Verification items for the finished model (mm, model axes). Coordinates: 2 decimals unless noted, no trailing zeros. Write each loop counter-clockwise with the first axis right and the second up, starting at its lowest first coordinate (ties: lowest second). Pieces come first, ordered by that corner, then holes. Notation, with made-up numbers: M 27,63.5 L 67,63.5 A34 cw 67,101.5 Z; hole C -20.75,41.25 d10. An arc over 180 degrees is marked long. Answer in a Markdown table with one row per item.
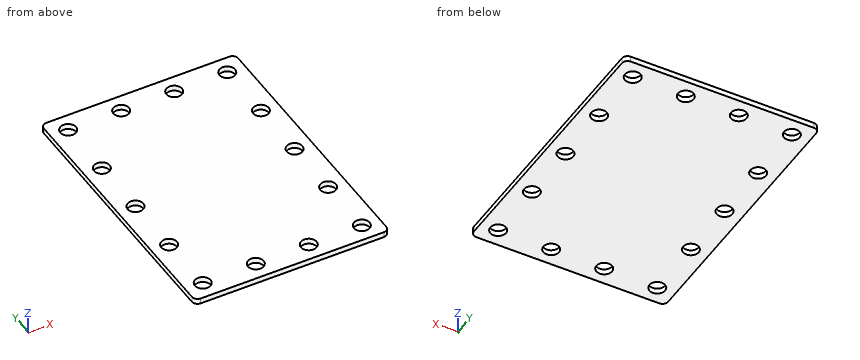
Autodesk Inventor part; units mm, degrees
ref_plane "YZ Plane" through (0, 0, 0) normal (1, 0, 0) x (0, 1, 0)
ref_plane "XZ Plane" through (0, 0, 0) normal (0, 1, 0) x (-1, 0, 0)
ref_plane "XY Plane" through (0, 0, 0) normal (0, 0, 1) x (1, 0, 0)
sketch "Sketch2" plane through (0, 0, 0) normal (0, 0, 1) x (1, 0, 0)
  line L0 (-55, -98) -> (55, -98)
  line L1 (55, -98) -> (55, 98)
  line L2 (55, 98) -> (-55, 98)
  line L3 (-55, 98) -> (-55, -98)
  line L4 (-55, -98) -> (55, 98) construction
  line L5 (55, -98) -> (-55, 98) construction
  line L6 (-105, -148) -> (105, -148)
  line L7 (105, -148) -> (105, 148)
  line L8 (105, 148) -> (-105, 148)
  line L9 (-105, 148) -> (-105, -148)
  point P0 (0, 0)
  dimension "d31" = 50
  dimension "d60" = 196
  dimension "d61" = 110
extrude "Plate2" add sketch "Sketch2" along normal blind 6 contours L3 L2 L1 L0 | L9 L8 L7 L6
sketch "Sketch5" plane through (0, 0, 6) normal (0, 0, 1) x (1, 0, 0)
  line L0 (105, -148) -> (-105, -148) construction
  line L1 (105, 148) -> (105, -148) construction
  line L2 (-105, 148) -> (105, 148) construction
  line L3 (-105, -148) -> (-105, 148) construction
  line L4 (-86, 129) -> (86, 129) construction
  line L5 (86, 129) -> (86, -129) construction
  line L6 (86, -129) -> (-86, -129) construction
  line L7 (-86, -129) -> (-86, 129) construction
  line L8 (-28.6667, -129) -> (28.6667, -129)
  line L9 (28.6667, -129) -> (28.6667, 129) construction
  line L10 (28.6667, 129) -> (-28.6667, 129)
  line L11 (-28.6667, 129) -> (-28.6667, -129) construction
  line L12 (-28.6667, 0) -> (28.6667, 0) construction
  point P0 (0, 0)
  point P1 (0, -129)
  point P2 (-86, -64.5)
  point P3 (-86, 0)
  point P4 (-86, 64.5)
  point P5 (86, 64.5)
  point P6 (86, 0)
  point P7 (86, -64.5)
  point P8 (0, 0)
  dimension "d34" = 19
  dimension "d47" = 64.5
  dimension "d48" = 64.5
  dimension "d49" = 57.3333
  dimension "d50" = 57.3333
fillet "Corner Round1" radius 6 4 edges at (-105, -148, 3) (-105, 148, 3) (105, 148, 3) (105, -148, 3)
hole "Hole1" at (-86, -129, 6) at (-86, -64.5, 6) at (-86, 0, 6) at (-86, 64.5, 6) at (-86, 129, 6) at (86, 129, 6) at (86, 64.5, 6) at (86, 0, 6) at (86, -64.5, 6) at (86, -129, 6) at (-28.6667, -129, 6) at (28.6667, 129, 6) at (28.6667, -129, 6) at (-28.6667, 129, 6) direction (0, 0, -1) diameter 17 end through all
equation "\"d60\" = ChargingHatch_width - 2 * Thickness"
equation "\"d61\" = ChargingHatch_hight - 2 * Thickness"
equation "\"d56\" = Thickness"
equation "\"d14\" = Thickness"
equation "\"BendReliefWidth\" = Thickness"
equation "\"BendReliefDepth\" = 0.5 * Thickness"
equation "\"CornerReliefSize\" = 4 * Thickness"
equation "\"MinimumRemnant\" = 2 * Thickness"
equation "\"TransitionRadius\" = BendRadius"
equation "\"JacobiRadiusSize\" = BendRadius"
equation "\"GapSize\" = Thickness"
properties part number "PRS 9607 charging flange rect_D1200" material "Steel"
1) Thickness scan on L1, parallel to Y at x = -29, z = 2.7; L2, parallel to X at y = 129, z = 2.2; L3, parallel to X at y = 64.5, z = 2. Record the ranges inside material, lowest first. Write a range as [from, to].
Response values:
| item | result |
|---|---|
| L1 | y = [-148, -137.49], [-120.51, 120.51], [137.49, 148] |
| L2 | x = [-105, -94.5], [-77.5, -37.17], [-20.17, 20.17], [37.17, 77.5], [94.5, 105] |
| L3 | x = [-105, -94.5], [-77.5, 77.5], [94.5, 105] |
2) Sectioned sample at A-A (y = -64.5). Record the cut outline in (x, z).
Response values:
| item | result |
|---|---|
| outline | M -105,0 L -94.5,0 L -94.5,6 L -105,6 Z; M -77.5,0 L 77.5,0 L 77.5,6 L -77.5,6 Z; M 94.5,0 L 105,0 L 105,6 L 94.5,6 Z |
3) Sectioned sample at D-D (x = 24.5). Record the cut outline in (y, z).
Response values:
| item | result |
|---|---|
| outline | M -148,0 L -136.41,0 L -136.41,6 L -148,6 Z; M -121.59,0 L 121.59,0 L 121.59,6 L -121.59,6 Z; M 136.41,0 L 148,0 L 148,6 L 136.41,6 Z |
4) Sectioned sample at C-C (y = -129). Record the cut outline in (x, z).
Response values:
| item | result |
|---|---|
| outline | M -105,0 L -94.5,0 L -94.5,6 L -105,6 Z; M -77.5,0 L -37.17,0 L -37.17,6 L -77.5,6 Z; M -20.17,0 L 20.17,0 L 20.17,6 L -20.17,6 Z; M 37.17,0 L 77.5,0 L 77.5,6 L 37.17,6 Z; M 94.5,0 L 105,0 L 105,6 L 94.5,6 Z |
5) Sectioned sample at B-B (x = 86). Record the cut outline in (y, z).
Response values:
| item | result |
|---|---|
| outline | M -148,0 L -137.5,0 L -137.5,6 L -148,6 Z; M -120.5,0 L -73,0 L -73,6 L -120.5,6 Z; M -56,0 L -8.5,0 L -8.5,6 L -56,6 Z; M 8.5,0 L 56,0 L 56,6 L 8.5,6 Z; M 73,0 L 120.5,0 L 120.5,6 L 73,6 Z; M 137.5,0 L 148,0 L 148,6 L 137.5,6 Z |
